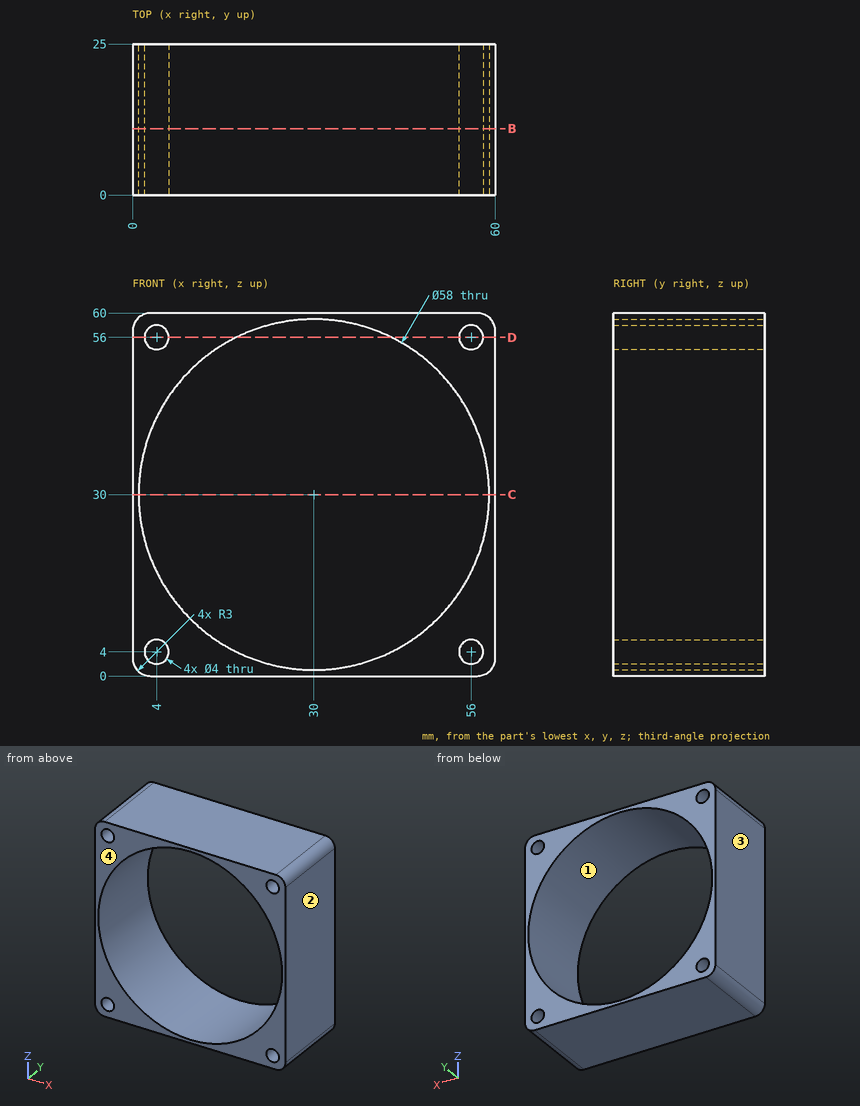
Check sheet for the drawn part. Datum: minimum x, y, z corner. Units: mm. Round coordinates to 2 decimals unless told otherwise and drop trailing zeros. Order: outer loops, then holes, each group sorted by start corner. A loop starts at its lowest first (then second) coordinate and runs counter-clockwise, first axis right, second up.
(1) Cross-section at B-B, the plane y = 11. Enter the section's corners in (x, z), and give its area (3 significant figures).
(2) Scan lines: probe 1 along Z at (x, y) = (3.5, 12); probe 2 along Z at (x, y) = (56, 5.25). Record each from-to range of solid material in increasing order.
(3) Cross-section at D-D, the plane z = 56. Enter the section's corners in (x, y).
(4) Draft check along X on the marked faces 1, 2, 3 and 4. Enter one of: pulls with the +X half, pulls with the -X half, needs draft (parallel to the pull), parting line crosses it, or undercut.
(5) Cross-section at C-C, the plane z = 30. Enter the section's corners in (x, y).
Check sheet entries:
1. outline: (0, 3) arc R3 ccw to (3, 0) - (57, 0) arc R3 ccw to (60, 3) - (60, 57) arc R3 ccw to (57, 60) - (3, 60) arc R3 ccw to (0, 57) - close; hole circle Ø58 at (30, 30); hole circle Ø4 at (4, 4); hole circle Ø4 at (4, 56); hole circle Ø4 at (56, 4); hole circle Ø4 at (56, 56)
1. area: 900 mm2
2. probe 1: z = 0 to 2.06, 5.94 to 18.22, 41.78 to 54.06, 57.94 to 60
2. probe 2: z = 0 to 2, 6 to 17.15, 42.85 to 54, 58 to 60
3. outline: (0, 0) - (2, 0) - (2, 25) - (0, 25) - close; (6, 0) - (17.15, 0) - (17.15, 25) - (6, 25) - close; (42.85, 0) - (54, 0) - (54, 25) - (42.85, 25) - close; (58, 0) - (60, 0) - (60, 25) - (58, 25) - close
4. face 1: undercut
4. face 2: pulls with the +X half
4. face 3: pulls with the -X half
4. face 4: needs draft
5. outline: (0, 0) - (1, 0) - (1, 25) - (0, 25) - close; (59, 0) - (60, 0) - (60, 25) - (59, 25) - close
